The model under review builds one solid part; all positions refer to its coordinate system, in mm. A direction names the side the tool comes from. Round coordinates to 2 decimals unless told otherwise and drop trailing zeros. Write each loop counter-clockwise with the first axis right and the second up, starting at its lowest first coordinate (ties: lowest second). Pieces come first, ordered by that corner, then holes. Notation, with made-up numbers: M 24,30 L 48,30 A9 ccw 48,40 Z; hole C 85,58.25 d11. An arc over 180 degrees is marked long. One line per item, written item: value. Start each with the question number.
1) Take a section at A-A, the plane x = 0. Write out the cut boundary in (y, z) (3 decimals), and give its area (3 significant figures).
2) For P1, Ø5, axis at x = -4, z = 2, coming from the -Y side; P2, Ø10, axis at y = 9.5, z = 4.5, coming from the -X side; P3, Ø6, axis at x = -2, z = -2.5, coming from the +Y side; P4, Ø1, axis at y = 34.5, z = 5, coming from the +X side, all flat-tipped, find the tip position at first contact; note any pin that passes through.
3) Take a section at D-D, the plane z = -8.5. Write out the cut boundary in (x, y).
4) Wall thickness on probe 1 along Z at (x, y) = (0, 28.5); probe 2 along Z at (x, y) = (0, 39.6): over which ranges is each line inside the solid? List them lowest first.
5) Take a section at C-C, the plane y = 32.5. Write out the cut boundary in (x, z).
6) Take a section at B-B, the plane z = 0. Write out the cut boundary in (x, y) (3 decimals), and give its area (3 significant figures).
7) Mouldability with a two-part tool opening along X and no side actions: class faces 1 (the face through (0, 0, -8.2)), 2 (the face through (-2, 39, -6)), 3 (the face through (-2.17, 21.2, -9.76)) as +X half, -X half, draft (parallel to the pull), parting line (faces both ways), or undercut.
8) Tool access review of faces 4 (the face through (0.6, 46, -7.4)), 5 (the face through (-1.73, 19.23, -7.81)), 6 (the face through (9, 43, 2)): name each direction out of +Z, -Z, +X, -X, +Y, -Y from which nothing blocks a thin tool from reaching the whole face with its end or side.
Autodesk Fusion 360 part; units mm, degrees
sketch "Sketch1" plane through (0, 0, 0) normal (0, 1, 0) x (1, 0, 0)
  circle A0 centre (0, 0) radius 10
  dimension "d1" = 20
extrude "Extrude1" add sketch "Sketch1" along normal blind 46
sketch "Sketch2" plane through (0, 0, 0) normal (0, 1, 0) x (1, 0, 0)
  circle A0 centre (0, 0) radius 8
  dimension "d4" = 16
extrude "Extrude2" cut sketch "Sketch2" along normal blind 39
sketch "Sketch3" plane through (0, 46, 0) normal (0, 1, 0) x (-1, 0, 0)
  circle A0 centre (0, 0) radius 10
  circle A1 centre (0, 0) radius 9
  dimension "d7" = 18
extrude "Extrude3" cut sketch "Sketch3" against normal blind 3
sketch "Sketch4" plane through (0, 46, 0) normal (0, 1, 0) x (-1, 0, 0)
  circle A0 centre (0, 0) radius 9
  circle A1 centre (0, 0) radius 7.265
  dimension "d10" = 14.53
extrude "Extrude4" cut sketch "Sketch4" against normal blind 6 contours A1
sketch "Sketch5" plane through (0, 40, 0) normal (0, 1, 0) x (-1, 0, 0)
  circle A0 centre (0, 0) radius 7.265
  circle A1 centre (0, 0) radius 6
  dimension "d13" = 12
extrude "Extrude5" cut sketch "Sketch5" against normal blind 10 contours A1
Checked values:
1. outline: M 0,-10 L 43,-10 L 43,-9 L 46,-9 L 46,-7.265 L 40,-7.265 L 40,-6 L 39,-6 L 39,-8 L 0,-8 Z; M 0,8 L 39,8 L 39,6 L 40,6 L 40,7.265 L 46,7.265 L 46,9 L 43,9 L 43,10 L 0,10 Z
1. area: 191 mm2
2. P1: stops at y = 39
2. P2: stops at x = -10
2. P3: stops at y = 40
2. P4: stops at x = 8.93
3. outline: M -5.27,0 L 5.27,0 L 5.27,43 L 2.96,43 L 2.96,46 L -2.96,46 L -2.96,43 L -5.27,43 Z
4. probe 1: z = -10 to -8, 8 to 10
4. probe 2: z = -10 to -6, 6 to 10
5. outline: C 0,0 d20; hole C 0,0 d16
6. outline: M -10,0 L -8,0 L -8,39 L -6,39 L -6,40 L -7.265,40 L -7.265,46 L -9,46 L -9,43 L -10,43 Z; M 6,39 L 8,39 L 8,0 L 10,0 L 10,43 L 9,43 L 9,46 L 7.265,46 L 7.265,40 L 6,40 Z
6. area: 191 mm2
7. face 1: draft
7. face 2: undercut
7. face 3: parting line
8. face 4: +Z, -Z, +X, -X, +Y
8. face 5: -Y
8. face 6: +Y
